Part model, mm, in its own coordinate system. Face numbers are marked on the shaded views. A direction names the side the tool comes from. Coordinates: 2 decimals unless noted, no trailing zeros. Loops run counter-clockwise (first coordinate to the right, second up) from the corner with the lowest first, then second, coordinate; pieces in that order, holes last. Notation, with made-up numbers: M -9,59 L 45,59 A10 ccw 45,78 Z; hole C -10.5,41 d6. An arc over 180 degrees is marked long. Use a Markdown table: item, result. Add a question column.
1) Pin check, flat tips, straight feed: pin 1 Ø5 at (x, y) = (21, -10) entering from +Z; pin 2 Ø6 at (x, y) = (50.5, -9) entering from +Z; pin 3 Ø1.5 at (x, z) = (24, -12.5) entering from +Y. Stop position of each tip, or through.
2) Tool access for the marked faces 1 and 2: list every direction of +Z, -Z, +X, -X, +Y, -Y with a clear straight run to the whole face (end or side of a thin tool).
3) Band-saw the part on A-A (x = 72). List the corners of the cut face in (y, z), plus the area to 3 significant figures.
4) Wall check: probe 1 along Y at (x, z) = (3.25, 0); probe 2 along X at (y, z) = (-18, 1); probe 3 along Z at (x, y) = (39.5, 0.5). Give the ranges that are in metal, low to high. Write a range as from..to.
from build123d import *

# Parameters (mm, degrees)
SKETCH_1_R             = 15
EXTRUDE_1_DEPTH        = 82
SKETCH_2_R             = 20
EXTRUDE_2_DEPTH        = 5
CHAMFER_1_SIZE         = 1
HOLE_WIZARD_M8_1_D     = 6.8
HOLE_WIZARD_M8_1_DEPTH = 15
HOLE_WIZARD_M8_1_TIP   = 2.042926105


with BuildPart() as part:
    # 草图1 → 凸台-拉伸1 (new body)
    with BuildSketch(Plane(origin=(0, 0, 0), x_dir=(0, 0, -1), z_dir=(1, 0, 0))):
        Circle(SKETCH_1_R)
    extrude(amount=EXTRUDE_1_DEPTH)

    # 草图2 → 凸台-拉伸2 (add)
    with BuildSketch(Plane(origin=(82, 0, 0), x_dir=(0, 0, -1), z_dir=(1, 0, 0))):
        Circle(SKETCH_2_R)
    extrude(amount=EXTRUDE_2_DEPTH)

    # 倒角1
    chamfer_1_edges = [part.edges().sort_by_distance(p)[0] for p in [
        (0, 0, 15),
        (87, 0, 20),
    ]]
    chamfer(chamfer_1_edges, length=CHAMFER_1_SIZE)

    # M8 螺纹孔的螺纹孔钻头1
    with Locations(Plane(origin=(0, 0, 0), x_dir=(0, 0, -1), z_dir=(-1, 0, 0))):
        with Locations((0, 0)):
            Hole(HOLE_WIZARD_M8_1_D / 2, depth=HOLE_WIZARD_M8_1_DEPTH)
            with Locations((0, 0, -(HOLE_WIZARD_M8_1_DEPTH + HOLE_WIZARD_M8_1_TIP / 2))):  # 118° drill point
                Cone(0, HOLE_WIZARD_M8_1_D / 2, HOLE_WIZARD_M8_1_TIP, mode=Mode.SUBTRACT)


solid = part.part
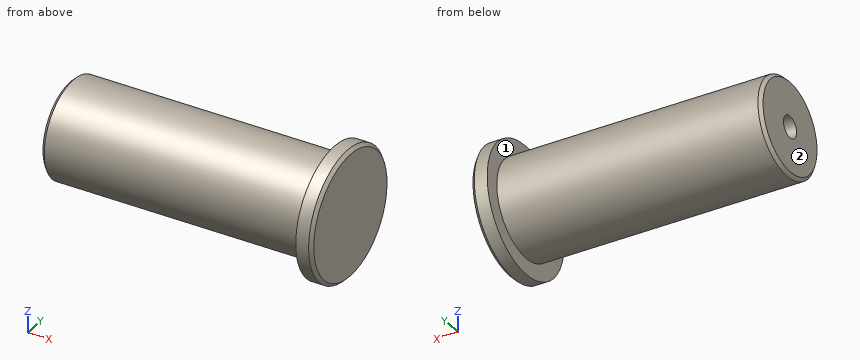
Entries:
| question | item | result |
|---|---|---|
| 1 | pin 1 | z = 12.99 |
| 1 | pin 2 | z = 13.75 |
| 1 | pin 3 | y = 9.32 |
| 2 | face 1 | -X |
| 2 | face 2 | +Z, -Z, -X, +Y, -Y |
| 3 | outline | C 0,0 d30 |
| 3 | area | 707 mm2 |
| 4 | probe 1 | -15..-3.4, 3.4..15 |
| 4 | probe 2 | 82..87 |
| 4 | probe 3 | -14.99..14.99 |
